For this review, take the finished solid that the model builds, in its own axes (mm). A direction names the side the tool comes from. Coordinates: 2 decimals unless noted, no trailing zeros. Loops run counter-clockwise (first coordinate to the right, second up) from the corner with the lowest first, then second, coordinate; pieces in that order, holes last. Notation, with made-up numbers: (-3, 4) - (26, 4) arc R32 ccw to (26, 30) - close; hole circle Ø8 at (59, -13.75). An arc over 180 degrees is marked (long way). One line per item, written item: value. Start each with the question number.
1. Take a section at B-B, the plane x = -0.5. State the section outline as (y, z) points (3 decimals), and give its area (3 significant figures).
2. To check wall thickness, follow line 1 (X direction, y = -1, z = 2.75); line 2 (X direction, y = 0.5, z = 8.5); line 3 (Z direction, x = 3, y = -3.5). State the ranges of each line that lie inside material, in increasing order. Write a range as from..to.
3. Take a section at C-C, the plane z = 1.75. State the section outline as (x, y) points, and give its area (3 significant figures).
4. Insertion check: pin 1 (5 mm diameter, centred on y = -3.5, z = 6.5, fed in from -X); pin 2 (9 mm diameter, centred on x = 0.5, y = 0.5, fed in from +Z); pin 3 (5 mm diameter, centred on y = -3.5, z = 6.5, fed in from +X). Each pin has a flat end and moves straight along its axis. Give the tip position at first contact, or say it passes through.
5. The part is to be moulded in two halves that separate along X. For faces 4 (the face through (-16.924, 0.381, 1.565)), 5 (the face through (21.844, 0, 2)), 6 (the face through (0, 7, 9.169)), say which applies: released by +X, released by -X, zero draft, split by the parting line, or undercut.
6. For faces 1 (the face through (-20, 0, 3.175)), 2 (the face through (0, 9, 3.175)), 3 (the face through (20, 0, 3.175)), list the 3-axis set-ups (+Z, -Z, +X, -X, +Y, -Y) from which the entire face can be reached by the end or side of a thin tool; tool diameter is ignored.
7. Take a section at A-A, the plane y = 0. Count the separate pieces of the cut face and the enclosed holes in it, and give its area (3 significant figures).
```python
from build123d import *

# Parameters (mm, degrees)
F0_W     = 43.688
F0_H     = 16.764
F0_R     = 1.27
F1_DEPTH = 3.175
F2_W     = 31.369
F2_H     = 20.0406
F3_DEPTH = 5.9944
F5_DEPTH = 0.254


with BuildPart() as f1:
    # F0 (on Top) → F1 (new body)
    with BuildSketch(Plane.XY):
        Rectangle(F0_W, F0_H)
        with Locations((-18.1356, 0)):
            Circle(F0_R, mode=Mode.SUBTRACT)
        with Locations((18.1356, 0)):
            Circle(F0_R, mode=Mode.SUBTRACT)
    extrude(amount=F1_DEPTH)

    # F2 (on face) → F3 (join)
    with BuildSketch(Plane.XY.offset(3.175)):
        Rectangle(F2_W, F2_H)
    extrude(amount=F3_DEPTH)

    # F4 (on face) → F5 (cut)
    with BuildSketch(Plane.XY.offset(9.1694)):
        Polygon((-11.8618, -5.588), (12.573, -5.588), (12.573, 5.588), (-11.861305, 5.588), (-11.861305, 2.286189), (-12.573, 2.286189), (-12.573, -2.286), (-11.8618, -2.286), align=None)
    extrude(amount=-F5_DEPTH, mode=Mode.SUBTRACT)


solid = f1.part
```
Solutions:
1. outline: (-10.02, 3.175) - (-8.382, 3.175) - (-8.382, 0) - (8.382, 0) - (8.382, 3.175) - (10.02, 3.175) - (10.02, 9.169) - (5.588, 9.169) - (5.588, 8.915) - (-5.588, 8.915) - (-5.588, 9.169) - (-10.02, 9.169) - close
1. area: 171 mm2
2. line 1: -21.84..-18.92, -17.35..17.35, 18.92..21.84
2. line 2: -15.68..15.68
2. line 3: 0..8.92
3. outline: (-21.84, -8.38) - (21.84, -8.38) - (21.84, 8.38) - (-21.84, 8.38) - close; hole circle Ø2.54 at (-18.14, 0); hole circle Ø2.54 at (18.14, 0)
3. area: 722 mm2
4. pin 1: x = -15.68
4. pin 2: z = 8.92
4. pin 3: x = 15.68
5. face 4: undercut
5. face 5: released by +X
5. face 6: zero draft
6. face 1: +Z, -X, +Y, -Y
6. face 2: -Z, +X, -X, +Y
6. face 3: +Z, +X, +Y, -Y
7. separate pieces: 3
7. enclosed holes: 0
7. area: 304 mm2
